CAD build for the part. Positions are in the model's coordinates, mm. A direction names the side the tool comes from. Round coordinates to 2 decimals unless told otherwise and drop trailing zeros. Order: outer loops, then holes, each group sorted by start corner. A loop starts at its lowest first (then second) coordinate and runs counter-clockwise, first axis right, second up. Notation, with made-up numbers: (69, -9.5) - (92, -9.5) arc R23 cw to (92, 16.5) - close; hole circle Ø11 at (86, 32.5). An arc over 180 degrees is marked (long way). Write item = value, one per line.
from build123d import *
from build123d.topology import SkipClean

# Parameters (mm, degrees)
SKETCH1_R             = 7
GEARPLATE_DEPTH       = 1.5
BOSS_EXTRUDE3_DEPTH   = 1.5
CIRPATTERN2_COUNT     = 12
SKETCH3_R             = 4.5
BACKPLATE_DEPTH       = 4
SKETCH4_R             = 7
PLATE_DEPTH           = 3
SKETCH6_R             = 11.5
ANGLEPLATE_DEPTH      = 2.5
ANGLEPLATE_DRAFT      = -35
SKETCH8_R             = 10.5
SMALLANGLEPLATE_DEPTH = 0.2
SMALLANGLEPLATE_DRAFT = 79
SKETCH9_R             = 7
DOMEEXTRUDE_DEPTH     = 0.5
DOME1_FACE_RADIUS     = 7
DOME1_HEIGHT          = 1.5
CUT_EXTRUDE1_DEPTH    = 3.8


with BuildPart() as part:
    # Sketch1 → GearPlate (new body)
    with BuildSketch(Plane.XY):
        Circle(SKETCH1_R)
    extrude(amount=GEARPLATE_DEPTH)

    # Sketch2 → Boss-Extrude3 (add)
    with BuildSketch(Plane.XY.offset(1.5)):
        with BuildLine():
            Line((-1.47374446, 6.843104359), (1.47374446, 6.843104359))
            add(Edge.make_bspline(
                [(-1.47374446, 6.843104359), (0, 13.556322037), (1.47374446, 6.843104359)],
                knots=[0, 0, 0, 1, 1, 1], degree=2))
        make_face()
    boss_extrude3 = extrude(amount=-BOSS_EXTRUDE3_DEPTH)

    # CirPattern2: Boss-Extrude3 ×12 about axis
    cirpattern2_axis = Axis((0, 0, 1.5), (0, 0, -1))
    for i in range(1, CIRPATTERN2_COUNT):
        add(boss_extrude3.rotate(cirpattern2_axis, i * 360 / CIRPATTERN2_COUNT))

    # Sketch3 → BackPlate (add)
    with BuildSketch(Plane(origin=(0, 0, 0), x_dir=(-1, 0, 0), z_dir=(0, 0, -1))):
        with Locations(Location((0, 0, 0), (0, 0, 180))):
            Circle(SKETCH3_R)
    extrude(amount=BACKPLATE_DEPTH)

    # Sketch4 → Plate (add)
    with BuildSketch(Plane.XY.offset(1.5)):
        with Locations(Location((0, 0, 0), (0, 0, 192.153701922))):
            Circle(SKETCH4_R)
    extrude(amount=PLATE_DEPTH)


with BuildPart() as angleplate_tool:
    # Sketch6 → AnglePlate (with draft: the straight prism first)
    with BuildSketch(Plane.XY.offset(7)):
        Circle(SKETCH6_R)
    extrude(amount=-ANGLEPLATE_DEPTH)
    # AnglePlate: the draft: its side faces are tilted about the plane it starts from
    angleplate_sides = [angleplate_tool.faces().sort_by_distance(p)[0] for p in [
        (-11.5, 0, 5.75),
    ]]
    draft(angleplate_sides, Plane.XY.offset(7), ANGLEPLATE_DRAFT)


with BuildPart() as part_1:
    add(part.part)

    # AnglePlate: add angleplate_tool
    add(angleplate_tool.part)


with BuildPart() as smallangleplate_tool:
    # Sketch8 → SmallAnglePlate (with draft: the straight prism first)
    with BuildSketch(Plane.XY.offset(7.2)):
        Circle(SKETCH8_R)
    extrude(amount=-SMALLANGLEPLATE_DEPTH)
    # SmallAnglePlate: the draft: its side faces are tilted about the plane it starts from
    smallangleplate_sides = [smallangleplate_tool.faces().sort_by_distance(p)[0] for p in [
        (-10.5, 0, 7.1),
    ]]
    draft(smallangleplate_sides, Plane.XY.offset(7.2), SMALLANGLEPLATE_DRAFT)


with BuildPart() as part_2:
    add(part_1.part)

    # SmallAnglePlate: add smallangleplate_tool
    add(smallangleplate_tool.part)

    # Sketch9 → DomeExtrude (add)
    with SkipClean():  # the faces are left unmerged after this step: merging them gives an invalid solid
        with BuildSketch(Plane.XY.offset(7.2)):
            with Locations(Location((0, 0, 0), (0, 0, 192.153701922))):
                Circle(SKETCH9_R)
        extrude(amount=DOMEEXTRUDE_DEPTH)

    # Dome1: a dome of height H over a round flat face of radius A is a cap of a sphere of radius (A * A + H * H) / (2 * H)
    dome1_r = (DOME1_FACE_RADIUS * DOME1_FACE_RADIUS + DOME1_HEIGHT * DOME1_HEIGHT) / (2 * DOME1_HEIGHT)
    dome1_base = Plane((0, 0, 7.7), z_dir=(0, 0, 1))
    with Locations(dome1_base.offset(DOME1_HEIGHT - dome1_r)):
        dome1_ball = Sphere(dome1_r, mode=Mode.PRIVATE)
    add(split(dome1_ball, bisect_by=dome1_base, keep=Keep.TOP, mode=Mode.PRIVATE))

    # Sketch11 → Cut-Extrude1 (cut)
    with SkipClean():  # the faces are left unmerged after this step: merging them gives an invalid solid
        with BuildSketch(Plane.XY.offset(12.2)):
            Polygon((-0.75, 2), (0.75, 2), (0.75, 0.75), (2, 0.75), (2, -0.75), (0.75, -0.75), (0.75, -2), (-0.75, -2), (-0.75, -0.75), (-2, -0.75), (-2, 0.75), (-0.75, 0.75), align=None)
        extrude(amount=-CUT_EXTRUDE1_DEPTH, mode=Mode.SUBTRACT)


solid = part_2.part
(1) Band-saw the part on B-B on z = 5. List the corners of the cut face in (x, y).
Solved:
outline = circle Ø20.2 at (0, 0)
(2) Band-saw the part on A-A on z = 3.5. List the corners of the cut face in (x, y), plus the area to 3 significant figures.
Solved:
outline = circle Ø14 at (0, 0)
area = 154 mm²
(3) Tool access for faces 4 (the flat face through (-7, -4, 1.5)), 5 (the flat face through (7, -4, 1.5)), 6 (the flat face through (-4, 7, 1.5)): list every direction of +Z, -Z, +X, -X, +Y, -Y with a clear straight run to the whole face (end or side of a thin tool).
Solved:
face_4 = -X, -Y
face_5 = +X, -Y
face_6 = -X, +Y
(4) Probe line 1 along Z through (x, y) = (-8, -1); line 2 along X through (y, z) = (1.25, 5.25); line 3 along Z through (x, y) = (-2.25, 9.25). List the from-to ranges inside material, lowest first.
Solved:
line_1 = 0 to 1.5, 4.5 to 7.2
line_2 = -10.2 to 10.2
line_3 = 4.5 to 7.2
(5) Pull direction Z, two halves, no side cores. Call faces 1 (the flat face through (-5, 0, 0)), 2 (the flat face through (-4, -7, 1.5)), 3 (the flat face through (2, -7, 7.2)): released by +Z, released by -Z, zero draft, split by the parting line, or undercut.
Solved:
face_1 = released by -Z
face_2 = undercut
face_3 = released by +Z
(6) Drop flat-ended pins along their axis: pin 1 (3.5 mm diameter, centred on x = 3.5, y = -7.5, fed in from +Z); pin 2 (2.5 mm diameter, centred on x = 0, y = 8.5, fed in from +Z); pin 3 (4 mm diameter, centred on x = 7, y = 2, fed in from -Z). Give the stop position or say it passes through.
Solved:
pin_1 = 7.9
pin_2 = 7.2
pin_3 = 0
